```python
from build123d import *

# Parameters (mm, degrees)
F0_W         = 85
F0_H         = 56
F1_DEPTH     = 1.6
F2_W         = 21.4
F2_H         = 16
F3_DEPTH     = 13.4
F4_W         = 17.2
F4_H         = 15.3
F5_DEPTH     = 16.4
F6_W         = 15
F6_H         = 11.6
F7_DEPTH     = 6.6
F8_W         = 7
F8_H         = 15
F9_DEPTH     = 6
F10_W        = 8
F10_H        = 5.7
F11_DEPTH    = 3
F12_W        = 17
F12_H        = 11
F13_DEPTH    = 1.5
F14_R        = 1.375
F15_DEPTH    = 3.101
F16_T1_DEPTH = 16.6
F16_T3_DEPTH = 9.1
F17_W        = 50.9
F17_H        = 5
F18_DEPTH    = 9
F20_DEPTH    = 2.4


# Not quite as in the source:
# - a fillet or chamfer that OpenCascade refuses, or shapes differently, is made with other operations: its cross-section is extruded or revolved along the edge and cut away or added


with BuildPart() as f1:
    # F0 (on Top) → F1 (new body)
    with BuildSketch(Plane.XY):
        Rectangle(F0_W, F0_H)
    extrude(amount=F1_DEPTH)

    # F2 (on face) → F3 (join)
    with BuildSketch(Plane.XY.offset(1.6)):
        with Locations((33.8, -17.75)):
            Rectangle(F2_W, F2_H)
    extrude(amount=F3_DEPTH)

    # F4 (on face) → F5 (join)
    with BuildSketch(Plane.XY.offset(1.6)):
        with Locations((35.9, 1)):
            Rectangle(F4_W, F4_H)
        with Locations((35.9, 19)):
            Rectangle(F4_W, F4_H)
    extrude(amount=F5_DEPTH)

    # F6 (on face) → F7 (join)
    with BuildSketch(Plane.XY.offset(1.6)):
        with Locations((-10.5, -23.2)):
            Rectangle(F6_W, F6_H)
    extrude(amount=F7_DEPTH)

    # F8 (on face) → F9 (join)
    with BuildSketch(Plane.XY.offset(1.6)):
        with Locations((11, -22.9)):
            Rectangle(F8_W, F8_H)
    extrude(amount=F9_DEPTH)

    # F10 (on face) → F11 (join)
    with BuildSketch(Plane.XY.offset(1.6)):
        with Locations((-31.9, -26.15)):
            Rectangle(F10_W, F10_H)
    extrude(amount=F11_DEPTH)

    # F12 (on face) → F13 (join)
    with BuildSketch(Plane(origin=(0, 0, 0), x_dir=(1, 0, 0), z_dir=(0, 0, -1))):
        with Locations((-37.7, 0)):
            Rectangle(F12_W, F12_H)
    extrude(amount=F13_DEPTH)

    # F14 (on face) → F15 (cut, through all)
    with BuildSketch(Plane.XY.offset(1.6)):
        with Locations((-39, -24.5)):
            Circle(F14_R)
        with Locations((19, -24.5)):
            Circle(F14_R)
        with Locations((-39, 24.5)):
            Circle(F14_R)
        with Locations((19, 24.5)):
            Circle(F14_R)
    extrude(amount=-F15_DEPTH, mode=Mode.SUBTRACT)

    # F16: fillet of radius 3 on 4 edges, made by hand

    # F16_s2 → F16_t1 (cut)
    with BuildSketch(Plane.XY.offset(-7.5)):
        with BuildLine():
            ThreePointArc((-39.5, -28), (-41.6213203436, -27.1213203436), (-42.5, -25))
            Line((-42.5, -25), (-42.5, -28))
            Line((-42.5, -28), (-39.5, -28))
        make_face()
        with BuildLine():
            ThreePointArc((-42.5, 25), (-41.6213203436, 27.1213203436), (-39.5, 28))
            Line((-39.5, 28), (-42.5, 28))
            Line((-42.5, 28), (-42.5, 25))
        make_face()
    extrude(amount=F16_T1_DEPTH, mode=Mode.SUBTRACT)

    # F16_s4 → F16_t3 (cut)
    with BuildSketch(Plane.XY.offset(-7.5)):
        with BuildLine():
            ThreePointArc((39.5, -28), (41.6213203436, -27.1213203436), (42.5, -25))
            Line((42.5, -25), (42.5, -28))
            Line((42.5, -28), (39.5, -28))
        make_face()
        with BuildLine():
            ThreePointArc((42.5, 25), (41.6213203436, 27.1213203436), (39.5, 28))
            Line((39.5, 28), (42.5, 28))
            Line((42.5, 28), (42.5, 25))
        make_face()
    extrude(amount=F16_T3_DEPTH, mode=Mode.SUBTRACT)

    # F17 (on face) → F18 (join)
    with BuildSketch(Plane.XY.offset(1.6)):
        with Locations((-10, 24.4839084893)):
            Rectangle(F17_W, F17_H)
    extrude(amount=F18_DEPTH)

    # F19 (on face) → F20 (cut)
    with BuildSketch(Plane.XZ.offset(30.4)):
        with BuildLine():
            ThreePointArc((11, 7.6), (13.1213203436, 6.7213203436), (14, 4.6))
            ThreePointArc((14, 4.6), (13.1213203436, 2.4786796564), (11, 1.6))
            Line((11, 1.6), (14.5, 1.6))
            Line((14.5, 1.6), (14.5, 7.6))
            Line((14.5, 7.6), (11, 7.6))
        make_face()
        with BuildLine():
            ThreePointArc((11, 1.6), (8, 4.6), (11, 7.6))
            Line((11, 7.6), (7.5, 7.6))
            Line((7.5, 7.6), (7.5, 1.6))
            Line((7.5, 1.6), (11, 1.6))
        make_face()
    extrude(amount=-F20_DEPTH, mode=Mode.SUBTRACT)


solid = f1.part
```
Build history of the part. All positions in model axes, mm. A direction names the side the tool comes from. Give positions to 0.01 mm unless a question says otherwise; leave off trailing zeros. Loops run counter-clockwise (first coordinate to the right, second up) from the corner with the lowest first, then second, coordinate; pieces in that order, holes last.
Item 1: Slice it at A-A, the plane x = 19. List the corners of the cut face in (y, z) (3 decimals).
Answers follow:
outline: (-28, 0) - (-25.875, 0) - (-25.875, 1.6) - (-28, 1.6) - close; (-23.125, 0) - (23.125, 0) - (23.125, 1.6) - (-23.125, 1.6) - close; (25.875, 0) - (28, 0) - (28, 1.6) - (25.875, 1.6) - close
Item 2: Slice it at D-D, the plane z = 2.5. Give the number of separate pieces and of enclosed holes in the cut face, and give its area (3 significant figures).
Answers follow:
separate pieces: 7
enclosed holes: 0
area: 1,440 mm2
Item 3: Which spindle directions (+Z, -Z, +X, -X, +Y, -Y) get a long thin tool onto all of the face, cutting with end or side? Do faces 1 (the face through (23.1, -18, 8)), 2 (the face through (41.64, 27.1, 0.79)), 3 (the face through (27.3, 19, 10)), 4 (the face through (36, 26.65, 10)). Say none if no direction does.
Answers follow:
face 1: +Z, +Y, -Y
face 2: -Z, +X, +Y
face 3: +Z, +Y
face 4: +Z, +X, +Y
Item 4: Slice it at B-B, the plane z = 14. List the corners of the cut face in (x, y).
Answers follow:
outline: (23.1, -25.75) - (44.5, -25.75) - (44.5, -9.75) - (23.1, -9.75) - close; (27.3, -6.65) - (44.5, -6.65) - (44.5, 8.65) - (27.3, 8.65) - close; (27.3, 11.35) - (44.5, 11.35) - (44.5, 26.65) - (27.3, 26.65) - close
Item 5: Flat gauge pins, fed straight in: pin 1 (5 mm diameter, centred on x = 35.5, z = 13, fed in from -Y); pin 2 (3 mm diameter, centred on x = -30, z = 9.5, fed in from -Y); pin 3 (10 mm diameter, centred on y = 4.5, z = 8.5, fed in from -X); pin 4 (1.6 mm diameter, centred on x = -39, y = 24.5, fed in from -Z). Where does each tip first touch, or does it go through?
Answers follow:
pin 1: stops at y = -25.75
pin 2: stops at y = 21.98
pin 3: stops at x = 27.3
pin 4: passes through
Item 6: Slice it at C-C, the plane x = 37. List the corners of the cut face in (y, z).
Answers follow:
outline: (-28, 0) - (28, 0) - (28, 1.6) - (26.65, 1.6) - (26.65, 18) - (11.35, 18) - (11.35, 1.6) - (8.65, 1.6) - (8.65, 18) - (-6.65, 18) - (-6.65, 1.6) - (-9.75, 1.6) - (-9.75, 15) - (-25.75, 15) - (-25.75, 1.6) - (-28, 1.6) - close
Item 7: Pull direction X, two halves, no side cores. Call faces 5 (the face through (-32, -29, 3)), 6 (the face through (15.45, 24, 6)), 7 (the face through (-18, -23, 5)), 8 (the face through (27.3, 1, 10)): released by +X, released by -X, zero draft, split by the parting line, or undercut.
Answers follow:
face 5: zero draft
face 6: undercut
face 7: undercut
face 8: released by -X
Item 8: Drill centre lines: line 1 (Y direction, x = 19, z = 0.5) (3 decimals); line 2 (Y direction, x = -34, z = 4.5); line 3 (Z direction, x = 8.5, y = 8). Where is each one in solid material? Low to high.
Answers follow:
line 1: y = -28 to -25.875, -23.125 to 23.125, 25.875 to 28
line 2: y = -29 to -23.3, 21.98 to 26.98
line 3: z = 0 to 1.6
